Check sheet for the modelled part. Datum: model origin and axes. Units: mm. Give positions to 0.01 mm unless a question says otherwise; leave off trailing zeros. Write each loop counter-clockwise with the first axis right and the second up, starting at its lowest first coordinate (ties: lowest second). Pieces come first, ordered by that corner, then holes. Notation, with made-up numbers: (13.5, 43.25) -> (18.5, 43.25) arc R18 ccw to (18.5, 66.25) -> close; hole circle Ø9 at (-29.5, 5). An arc over 180 degrees is marked (long way). Use a Markdown table: item, result. Add a question column.
1. Cross-section at B-B (x = -86). Enter the section's corners in (y, z), then the cut area to 3 significant figures.
2. Cross-section at C-C (z = 69.5). Enter the section's corners in (x, y).
3. Cross-section at A-A (y = -1.5). Enter the section's corners in (x, z), then the cut area to 3 significant figures.
4. Scan lines: probe 1 along X at (y, z) = (-2, -79); probe 2 along Z at (x, y) = (-90.5, -0.5); probe 3 along X at (y, z) = (1.5, -64). Record each from-to range of solid material in increasing order. Write a range as [from, to].
from build123d import *

# Parameters (mm, degrees)
ESBO_O1_W                = 200
ESBO_O1_H                = 180
RESSALTO_EXTRUS_O1_DEPTH = 3
CHANFRO1_SIZE            = 30


with BuildPart() as part:
    # Esboço1 → Ressalto-extrusão1 (new, symmetric)
    with BuildSketch(Plane(origin=(0, 0, 0), x_dir=(1, 0, 0), z_dir=(0, 1, 0))):
        Rectangle(ESBO_O1_W, ESBO_O1_H)
    extrude(amount=RESSALTO_EXTRUS_O1_DEPTH, both=True)

    # Chanfro1
    chanfro1_edges = [part.edges().sort_by_distance(p)[0] for p in [
        (100, 0, 90),
        (-100, 0, 90),
        (-100, 0, -90),
        (100, 0, -90),
    ]]
    chamfer(chanfro1_edges, length=CHANFRO1_SIZE)


solid = part.part
Worked answers:
| question | item | result |
|---|---|---|
| 1 | outline | (-3, -74) -> (3, -74) -> (3, 74) -> (-3, 74) -> close |
| 1 | area | 888 mm² |
| 2 | outline | (-90.5, -3) -> (90.5, -3) -> (90.5, 3) -> (-90.5, 3) -> close |
| 3 | outline | (-100, -60) -> (-70, -90) -> (70, -90) -> (100, -60) -> (100, 60) -> (70, 90) -> (-70, 90) -> (-100, 60) -> close |
| 3 | area | 34,200 mm² |
| 4 | probe 1 | x = [-81, 81] |
| 4 | probe 2 | z = [-69.5, 69.5] |
| 4 | probe 3 | x = [-96, 96] |
